Autodesk Inventor part; units mm, degrees
ref_plane "Work Plane1" through (0, -20, 0) normal (0, -1, 0) x (1, 0, 0)
ref_plane "YZ Plane" through (0, 0, 0) normal (1, 0, 0) x (0, 1, 0)
ref_plane "XZ Plane" through (0, 0, 0) normal (0, 1, 0) x (-1, 0, 0)
sketch "Sketch1" plane through (0, 0, 0) normal (1, 0, 0) x (0, 1, 0)
  arc A0 (0, -20) -> (0, 20) centre (0, 0) ccw
  arc A1 (0, -9) -> (0, 9) centre (0, 0) ccw
  line L0 (0, 20) -> (0, 9)
  line L1 (0, -9) -> (0, -20)
  dimension "d0" = 18
  dimension "d1" = 40
  dimension "d10" = 11
  dimension "d11" = 11
extrude "Extrusion1" add sketch "Sketch1" along normal blind 15.5
ref_plane "Work Plane1" through (0, -20, 0) normal (0, -1, 0) x (1, 0, 0)
sketch "Sketch2" plane through (0, -20, 0) normal (0, -1, 0) x (1, 0, 0)
  line L0 (0, 20) -> (0, 9)
  line L1 (0, 9) -> (15.5, 9)
  line L2 (15.5, 20) -> (15.5, 9)
  line L3 (0, 20) -> (15.5, 20)
  line L4 (0, -9) -> (0, -20)
  line L5 (0, -20) -> (15.5, -20)
  line L6 (15.5, -9) -> (15.5, -20)
  line L7 (0, -9) -> (15.5, -9)
  circle A0 centre (7.75, 14.5) radius 2
  circle A1 centre (7.75, -14.5) radius 2
  line L8 (15.5, 14.5) -> (0, 14.5) construction
  line L9 (7.75, 9) -> (7.75, 20) construction
  line L10 (7.75, -9) -> (7.75, -20) construction
  line L11 (0, -14.5) -> (15.5, -14.5) construction
  point P0 (0, 0)
  dimension "d6" = 4
  dimension "d7" = 4
extrude "Extrusion2" cut sketch "Sketch2" against normal through all contours A0 | A1
equation "\"d7\" = d6"
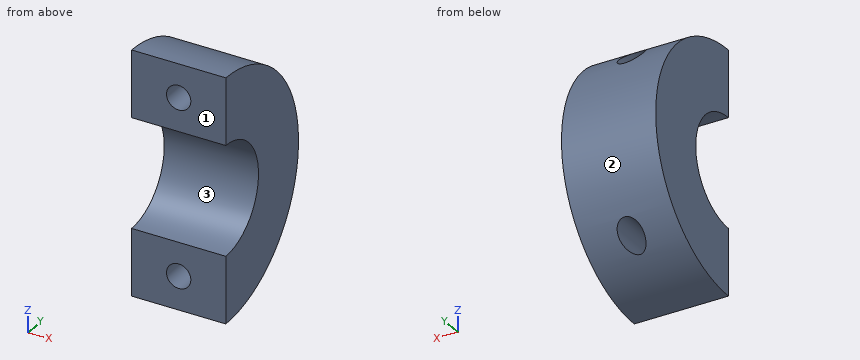
Could you check a few things on this model? Use its own coordinates, in mm. Face numbers are marked on the shaded views. Give positions to 0.01 mm unless a question says otherwise; leave off trailing zeros. Order: outer loops, then holes, each group sorted by start corner. A loop starts at its lowest first (then second) coordinate and runs counter-clockwise, first axis right, second up.
Item 1: If we section it at C-C, the plane x = 7.75: Write out the boundary of the cut face in (y, z), plus the area to 3 significant figures.
Item 2: I need wall thicknesses on line 1 (X direction, y = 7.75, z = 14.5); line 2 (Z direction, x = 9, y = 11.5); line 3 (Z direction, x = 7.75, y = 5). Which ranges of each line are inside material? Lowest first, please.
Item 3: If we section it at B-B, the plane z = -14.5: Write out the boundary of the cut face in (x, y), plus the area to 3 significant figures.
Item 4: If we section it at A-A, the plane y = 3: Write out the boundary of the cut face in (x, z), plus the area to 3 significant figures.
Item 5: I'm going to push flat-ended pins straight in: pin 1 (1.5 mm diameter, centred on x = 7, z = 6, fed in from +Y); pin 2 (1 mm diameter, centred on x = 7, z = -3.5, fed in from -Y); pin 3 (6.5 mm diameter, centred on x = 7.75, z = 14.5, fed in from +Y); pin 4 (3.5 mm diameter, centred on x = 7.75, z = -14.5, fed in from +Y). Where does each tip first touch, or does it pass through?
Item 6: If we section it at D-D, the plane x = 5: Write out the boundary of the cut face in (y, z).
Item 7: If we mould it in two halves opening along Z, with no side actions, what happens to the marked faces 1, 2 and 3? For each: pulls with the +Z half, pulls with the -Z half, needs draft (parallel to the pull), parting line crosses it, or undercut.
Values:
1. outline: (0, -20) arc R20 ccw to (11.3, -16.5) - (0, -16.5) - close; (0, -12.5) - (15.61, -12.5) arc R20 ccw to (15.61, 12.5) - (0, 12.5) - (0, 9) arc R9 cw to (0, -9) - close; (0, 16.5) - (11.3, 16.5) arc R20 ccw to (0, 20) - close
1. area: 392 mm2
2. line 1: x = 0 to 5.75, 9.75 to 15.5
2. line 2: z = -16.36 to -16.06, -12.94 to 12.94, 16.06 to 16.36
2. line 3: z = -19.36 to -16.5, -12.5 to -7.48, 7.48 to 12.5, 16.5 to 19.36
3. outline: (0, 0) - (5.75, 0) - (5.75, 13.77) - (0, 13.77) - close; (9.75, 0) - (15.5, 0) - (15.5, 13.77) - (9.75, 13.77) - close
3. area: 158 mm2
4. outline: (0, -19.77) - (15.5, -19.77) - (15.5, -8.49) - (0, -8.49) - close; (0, 8.49) - (15.5, 8.49) - (15.5, 19.77) - (0, 19.77) - close; hole circle Ø4 at (7.75, -14.5); hole circle Ø4 at (7.75, 14.5)
4. area: 325 mm2
5. pin 1: stops at y = 19.3
5. pin 2: stops at y = 8.06
5. pin 3: stops at y = 16.54
5. pin 4: passes through
6. outline: (0, -20) arc R20 ccw to (0, 20) - (0, 9) arc R9 cw to (0, -9) - close
7. face 1: needs draft
7. face 2: parting line crosses it
7. face 3: undercut
